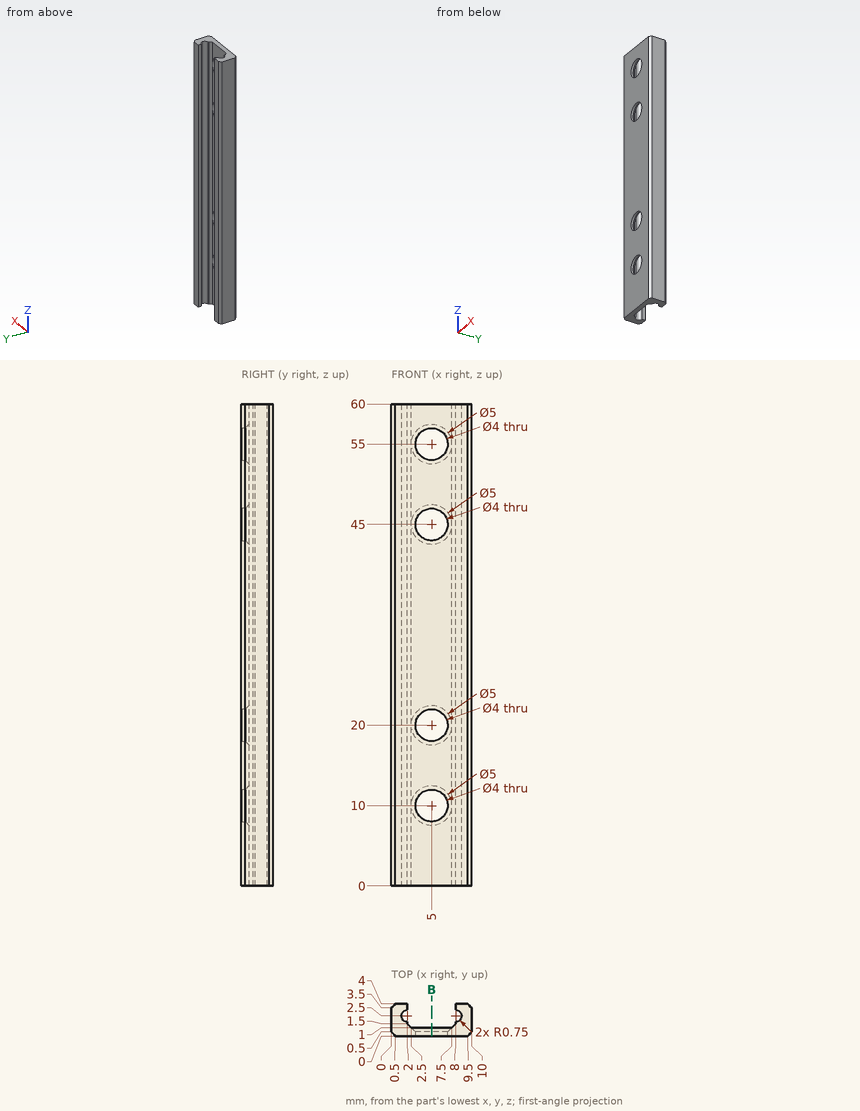
Check sheet for the drawn part. Datum: minimum x, y, z corner. Units: mm. Round coordinates to 2 decimals unless told otherwise and drop trailing zeros. Order: outer loops, then holes, each group sorted by start corner. A loop starts at its lowest first (then second) coordinate and runs counter-clockwise, first axis right, second up. Notation, with made-up numbers: M -31.75,-21 L 25.25,-21 A34 ccw 25.25,15 Z; hole C 41,89.5 d9. An arc over 180 degrees is marked long. Write each question's results on one line, items separated by ' | '. Start each with the question number.
1. Go/stop test with flat-tipped pins: P1, Ø3.5, axis at x = 5, z = 55, coming from the -Y side; P2, Ø4.5, axis at x = 5, z = 45, coming from the -Y side. Record where each tip stops, or that it passes through.
2. Cross-section at B-B on x = 5. Record the boundary of the cut face in (y, z).
3. Material ranges on L1, parallel to X at y = 2.4, z = 27; L2, parallel to Y at x = 7.75, z = 57.5; L3, parallel to X at y = 3.3, z = 11, recorded low to high. Write a range as from..to.
Resolved:
1) P1: through | P2: y = 0
2) outline: M 0,0 L 1,0 L 1,7.5 L 0.5,8 L 0,8 Z; M 0,12 L 0.5,12 L 1,12.5 L 1,17.5 L 0.5,18 L 0,18 Z; M 0,22 L 0.5,22 L 1,22.5 L 1,42.5 L 0.5,43 L 0,43 Z; M 0,47 L 0.5,47 L 1,47.5 L 1,52.5 L 0.5,53 L 0,53 Z; M 0,57 L 0.5,57 L 1,57.5 L 1,60 L 0,60 Z
3) L1: 0..1.26, 8.74..10 | L2: 0..1.25 | L3: 0..2, 8..10
